Drawing for the job (mm, zero at the part's lowest x, y, z). A direction names the side the tool comes from. Coordinates: 2 decimals unless noted, no trailing zeros. Loops run counter-clockwise (first coordinate to the right, second up) from the corner with the lowest first, then second, coordinate; pieces in that order, holes last. Notation, with made-up numbers: (-28.5, 17.5) - (11.5, 17.5) arc R14 cw to (11.5, 24.5) - close; hole circle Ø3 at (85, 6). An arc over 180 degrees is marked (long way). One line per item, written item: value.
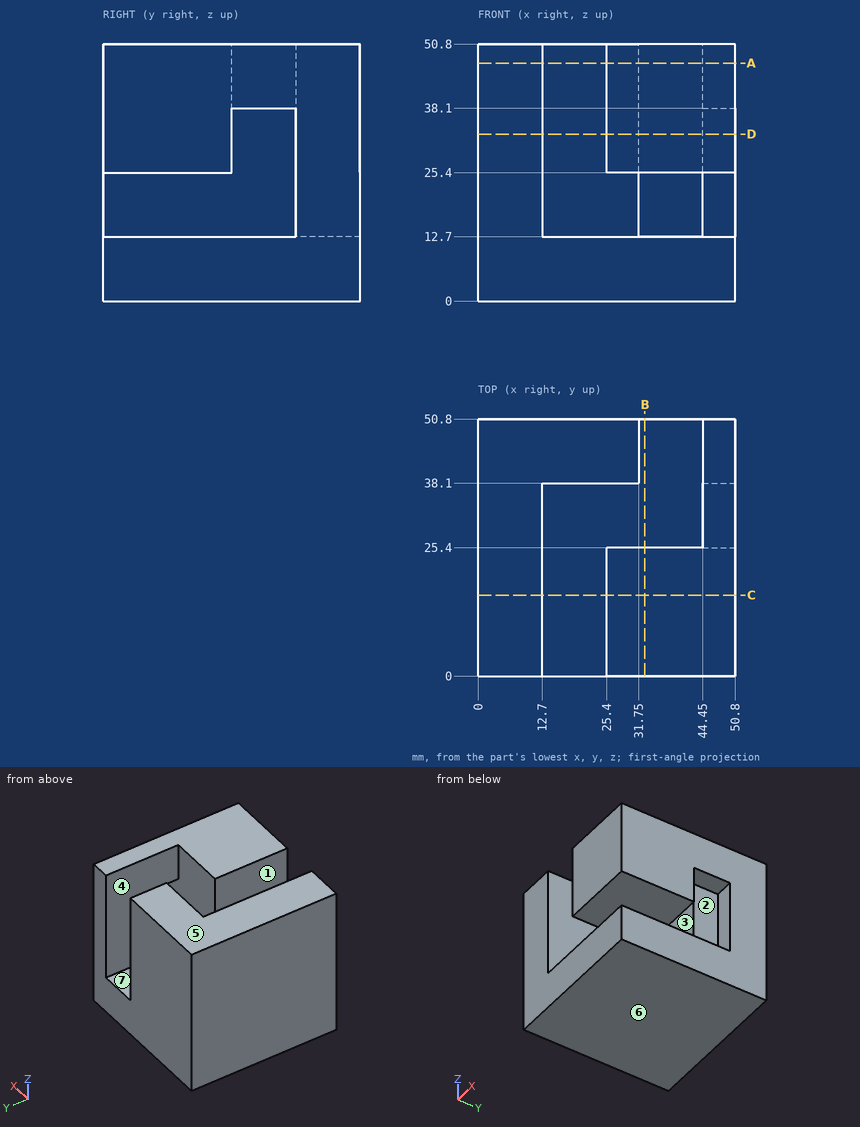
Item 1: Cut at C-C, the plane y = 16. Write the cut outline in (x, z).
Check result:
outline: (0, 0) - (50.8, 0) - (50.8, 12.7) - (12.7, 12.7) - (12.7, 50.8) - (0, 50.8) - close; (25.4, 25.4) - (50.8, 25.4) - (50.8, 50.8) - (25.4, 50.8) - close
Item 2: Tool access for the marked faces 1, 2 and 3: list every direction of +Z, -Z, +X, -X, +Y, -Y with a clear straight run to the whole face (end or side of a thin tool).
Check result:
face 1: +Z, -Y
face 2: +Z, +Y
face 3: +Z
Item 3: Cut at D-D, the plane z = 33. Write the cut outline in (x, y).
Check result:
outline: (0, 0) - (12.7, 0) - (12.7, 38.1) - (31.75, 38.1) - (31.75, 50.8) - (0, 50.8) - close; (25.4, 0) - (50.8, 0) - (50.8, 25.4) - (25.4, 25.4) - close; (44.45, 38.1) - (50.8, 38.1) - (50.8, 50.8) - (44.45, 50.8) - close
Item 4: Cut at B-B, the plane x = 33. Write the cut outline in (y, z).
Check result:
outline: (0, 0) - (50.8, 0) - (50.8, 12.7) - (0, 12.7) - close; (0, 25.4) - (25.4, 25.4) - (25.4, 50.8) - (0, 50.8) - close
Item 5: Pull direction Z, two halves, no side cores. Call the marked faces 4, 5, 6 and 7: released by +Z, released by -Z, zero draft, split by the parting line, or undercut.
Check result:
face 4: zero draft
face 5: released by +Z
face 6: released by -Z
face 7: undercut
Item 6: Cut at A-A, the plane z = 47. Write the cut outline in (x, y), then the cut area to 3 significant figures.
Check result:
outline: (0, 0) - (12.7, 0) - (12.7, 38.1) - (31.75, 38.1) - (31.75, 50.8) - (0, 50.8) - close; (25.4, 0) - (50.8, 0) - (50.8, 50.8) - (44.45, 50.8) - (44.45, 25.4) - (25.4, 25.4) - close
area: 1,690 mm^2
Item 7: Probe probe 1 along Z at (x, y) = (28, 24.5); probe 2 along X at (y, z) = (44.5, 40). List the from-to ranges inside material, lowest first. Write a range as from..to.
Check result:
probe 1: z = 0..12.7, 25.4..50.8
probe 2: x = 0..31.75, 44.45..50.8
